The listing builds one solid part. Answer for the finished solid, in the listing's coordinates (mm). A direction names the side the tool comes from. Round coordinates to 2 decimals unless told otherwise and drop trailing zeros. Use a Markdown table: item, result. Add a question column.
1) Find the intervals of material crossed by probe 1 along X at (y, z) = (12, 7.75); probe 2 along X at (y, z) = (-13, 15); probe 3 along Y at (x, z) = (-18, 2.75), in increasing order. Write a range as from..to.
2) Determine the mould class of faces 5 (the flat face through (-38.04, -24.13, 2.87)), 6 (the flat face through (-0.2, 25.3, 20)), 7 (the flat face through (-11.64, 18.17, 9.86)) for opening direction Y: +Y half, -Y half, draft (parallel to the pull), parting line (faces both ways), or undercut.
3) A tool of negligible diameter and unlimited length cuts with its end or side. For faces 1 (the flat face through (-22.64, -8.02, 21.48)), 2 (the flat face through (0, -25.009, 10)), 3 (the flat face through (28, -5, 20)), 4 (the flat face through (16.98, -14.62, 21.48)), from which of +Z, -Z, +X, -X, +Y, -Y can it reach the whole face along a straight path? Write none if from no direction.
4) A cutting plane is placed at A-A (z = 8.75). State how many separate pieces and enclosed holes the cut face has, then the cut area to 3 significant figures.
5) Each of these flat-tipped pins is pushed along its axis until it touches: P1, Ø4, axis at y = -20, z = 9, coming from the +X side; P2, Ø6.5, axis at x = -3.5, y = -14, coming from the +Z side. Where does it stop, or does it pass through?
```python
from build123d import *

# Parameters (mm, degrees)
F1_DEPTH      = 20
F2_R          = 7
F3_DEPTH      = 98.6163846154
F3_DEPTH_BACK = 8.6163846154
F4_R          = 7
F5_DEPTH      = 98.6163846154
F5_DEPTH_BACK = 8.6163846154
F7_DEPTH      = 3
F8_T4_DEPTH   = 57.4298435113
F8_T9_DEPTH   = 57.4298435113
F8_T14_DEPTH  = 56.5459149398
F8_T19_DEPTH  = 56.5459149398
F8_T24_DEPTH  = 56.5459149398
F8_T29_DEPTH  = 56.5459149398
F8_T34_DEPTH  = 57.4298435113
F8_T39_DEPTH  = 57.4298435113
F9_T1_DEPTH   = 31.2168298797
F9_T3_DEPTH   = 31.2168298797
F9_T5_DEPTH   = 31.2168298797
F10_R         = 3


# Not quite as in the source:
# - a fillet or chamfer that OpenCascade refuses, or shapes differently, is made with other operations: its cross-section is extruded or revolved along the edge and cut away or added


with BuildPart() as f1:
    # F0 (on Top) → F1 (new body)
    with BuildSketch(Plane.XY):
        Polygon((-23.609552012, 25.0086836473), (0, 25.0086836473), (23.609552012, 25.0086836473), (34.109552012, 31.0086836473), (-34.109552012, 31.0086836473), align=None)
        Polygon((0, 11.517511069), (-23.609552012, 25.0086836473), (-34.109552012, 31.0086836473), (-44.0323307792, 13.6438208048), (-38.0323307792, 10.2152493762), (-20.1556443707, 0), align=None)
        Polygon((34.109552012, 31.0086836473), (23.609552012, 25.0086836473), (0, 11.517511069), (20.1556443707, 0), (38.0323307792, 10.2152493762), (44.0323307792, 13.6438208048), align=None)
        Polygon((-38.0323307792, 10.2152493762), (-44.0323307792, 13.6438208048), (-44.0323307792, -13.6438208048), (-38.0323307792, -10.2152493762), (-38.0323307792, 0), align=None)
        Polygon((0, -11.517511069), (-20.1556443707, 0), (-38.0323307792, -10.2152493762), (-44.0323307792, -13.6438208048), (-34.109552012, -31.0086836473), (-23.609552012, -25.0086836473), align=None)
        Polygon((38.0323307792, -10.2152493762), (20.1556443707, 0), (0, -11.517511069), (23.609552012, -25.0086836473), (34.109552012, -31.0086836473), (44.0323307792, -13.6438208048), align=None)
        Polygon((44.0323307792, -13.6438208048), (44.0323307792, 13.6438208048), (38.0323307792, 10.2152493762), (38.0323307792, 0), (38.0323307792, -10.2152493762), align=None)
        Polygon((-23.609552012, -25.0086836473), (-34.109552012, -31.0086836473), (34.109552012, -31.0086836473), (23.609552012, -25.0086836473), (0, -25.0086836473), align=None)
        Polygon((20.1556443707, 0), (0, 11.517511069), (-20.1556443707, 0), (0, -11.517511069), align=None)
    extrude(amount=F1_DEPTH)

    # F2 (on face) → F3 (cut, two sides)
    with BuildSketch(Plane(origin=(-39.0709413956, -22.3262522261, 0), x_dir=(0.4961389384, -0.8682431421, 0), z_dir=(-0.8682431421, -0.4961389384, 0))) as f3_sk:
        with Locations((0, 10)):
            Circle(F2_R)
    extrude(amount=-F3_DEPTH, mode=Mode.SUBTRACT)
    extrude(f3_sk.sketch, amount=F3_DEPTH_BACK, mode=Mode.SUBTRACT)

    # F4 (on face) → F5 (cut, two sides)
    with BuildSketch(Plane(origin=(39.0709413956, -22.3262522261, 0), x_dir=(0.4961389384, 0.8682431421, 0), z_dir=(0.8682431421, -0.4961389384, 0))) as f5_sk:
        with Locations((0, 10)):
            Circle(F4_R)
    extrude(amount=-F5_DEPTH, mode=Mode.SUBTRACT)
    extrude(f5_sk.sketch, amount=F5_DEPTH_BACK, mode=Mode.SUBTRACT)

    # F6 (on face) → F7 (join)
    with BuildSketch(Plane.XY.offset(20)):
        Polygon((0, 0.8638133302), (-38.6988371918, 22.9774345827), (-39.0709413956, 22.3262522261), (-39.4430455994, 21.6750698695), (-1.5116733278, 0), align=None)
        Polygon((38.6988371918, 22.9774345827), (0, 0.8638133302), (1.5116733278, 0), (39.4430455994, 21.6750698695), (39.0709413956, 22.3262522261), align=None)
        Polygon((1.5116733278, 0), (0, 0.8638133302), (-1.5116733278, 0), (0, -0.8638133302), align=None)
        Polygon((39.4430455994, -21.6750698695), (1.5116733278, 0), (0, -0.8638133302), (38.6988371918, -22.9774345827), (39.0709413956, -22.3262522261), align=None)
        Polygon((0, -0.8638133302), (-1.5116733278, 0), (-39.4430455994, -21.6750698695), (-39.0709413956, -22.3262522261), (-38.6988371918, -22.9774345827), align=None)
    extrude(amount=F7_DEPTH)

    # F8: chamfer of 5 on 8 edges, made by hand


with BuildPart() as f8_tool2:
    # F8_s3 → F8_t4 (new body)
    with BuildSketch(Plane(origin=(-39.0709413956, -22.3262522261, 0), x_dir=(0, 0, 1), z_dir=(0.8682431421, 0.4961389384, 0))):
        Polygon((20, 5.75), (25, 0.75), (20, 0.75), align=None)
    extrude(amount=F8_T4_DEPTH)

    split(bisect_by=Plane.XY.offset(23), keep=Keep.BOTTOM)


with BuildPart() as f1_1:
    add(f1.part)

    # F8_t1: union F8_tool2
    add(f8_tool2.part)


with BuildPart() as f8_tool7:
    # F8_s8 → F8_t9 (new body)
    with BuildSketch(Plane(origin=(-10.7921263863, 6.1669293636, 0), x_dir=(0, 0, 1), z_dir=(0.8682431421, -0.4961389384, 0))):
        Polygon((20, 5.75), (25, 0.75), (20, 0.75), align=None)
    extrude(amount=F8_T9_DEPTH)

    split(bisect_by=Plane.XY.offset(23), keep=Keep.BOTTOM)


with BuildPart() as f1_2:
    add(f1_1.part)

    # F8_t6: union F8_tool7
    add(f8_tool7.part)


with BuildPart() as f8_tool12:
    # F8_s13 → F8_t14 (new body)
    with BuildSketch(Plane(origin=(10.0246614661, 5.7283779806, 0), x_dir=(0, 0, 1), z_dir=(-0.8682431421, -0.4961389384, 0))):
        Polygon((20, 5.75), (25, 0.75), (20, 0.75), align=None)
    extrude(amount=F8_T14_DEPTH)

    split(bisect_by=Plane.XY.offset(23), keep=Keep.BOTTOM)


with BuildPart() as f1_3:
    add(f1_2.part)

    # F8_t11: union F8_tool12
    add(f8_tool12.part)


with BuildPart() as f8_tool17:
    # F8_s18 → F8_t19 (new body)
    with BuildSketch(Plane(origin=(-39.0709413956, 22.3262522261, 0), x_dir=(0, 0, 1), z_dir=(0.8682431421, -0.4961389384, 0))):
        Polygon((20, 5.75), (25, 0.75), (20, 0.75), align=None)
    extrude(amount=F8_T19_DEPTH)

    split(bisect_by=Plane.XY.offset(23), keep=Keep.BOTTOM)


with BuildPart() as f1_4:
    add(f1_3.part)

    # F8_t16: union F8_tool17
    add(f8_tool17.part)


with BuildPart() as f8_tool22:
    # F8_s23 → F8_t24 (new body)
    with BuildSketch(Plane(origin=(39.0709413956, -22.3262522261, 0), x_dir=(0, 0, 1), z_dir=(-0.8682431421, 0.4961389384, 0))):
        Polygon((20, 5.75), (25, 0.75), (20, 0.75), align=None)
    extrude(amount=F8_T24_DEPTH)

    split(bisect_by=Plane.XY.offset(23), keep=Keep.BOTTOM)


with BuildPart() as f1_5:
    add(f1_4.part)

    # F8_t21: union F8_tool22
    add(f8_tool22.part)


with BuildPart() as f8_tool27:
    # F8_s28 → F8_t29 (new body)
    with BuildSketch(Plane(origin=(-10.0246614661, -5.7283779806, 0), x_dir=(0, 0, 1), z_dir=(0.8682431421, 0.4961389384, 0))):
        Polygon((20, 5.75), (25, 0.75), (20, 0.75), align=None)
    extrude(amount=F8_T29_DEPTH)

    split(bisect_by=Plane.XY.offset(23), keep=Keep.BOTTOM)


with BuildPart() as f1_6:
    add(f1_5.part)

    # F8_t26: union F8_tool27
    add(f8_tool27.part)


with BuildPart() as f8_tool32:
    # F8_s33 → F8_t34 (new body)
    with BuildSketch(Plane(origin=(10.7921263863, -6.1669293636, 0), x_dir=(0, 0, 1), z_dir=(-0.8682431421, 0.4961389384, 0))):
        Polygon((20, 5.75), (25, 0.75), (20, 0.75), align=None)
    extrude(amount=F8_T34_DEPTH)

    split(bisect_by=Plane.XY.offset(23), keep=Keep.BOTTOM)


with BuildPart() as f1_7:
    add(f1_6.part)

    # F8_t31: union F8_tool32
    add(f8_tool32.part)


with BuildPart() as f8_tool37:
    # F8_s38 → F8_t39 (new body)
    with BuildSketch(Plane(origin=(39.0709413956, 22.3262522261, 0), x_dir=(0, 0, 1), z_dir=(-0.8682431421, -0.4961389384, 0))):
        Polygon((20, 5.75), (25, 0.75), (20, 0.75), align=None)
    extrude(amount=F8_T39_DEPTH)

    split(bisect_by=Plane.XY.offset(23), keep=Keep.BOTTOM)


with BuildPart() as f1_8:
    add(f1_7.part)

    # F8_t36: union F8_tool37
    add(f8_tool37.part)

    # F9: chamfer of 5 on 4 edges, made by hand

    # F9_s2 → F9_t1 (cut)
    with BuildSketch(Plane(origin=(7.7439424177, -13.5518992309, 0), x_dir=(0, 0, 1), z_dir=(-0.4961389384, 0.8682431421, 0))):
        Polygon((18, -45), (23, -40), (23, -45), align=None)
        Polygon((18, 45), (23, 40), (23, 45), align=None)
    extrude(amount=F9_T1_DEPTH, mode=Mode.SUBTRACT)

    # F9_s4 → F9_t3 (cut)
    with BuildSketch(Plane(origin=(7.7439424177, 13.5518992309, 0), x_dir=(0, 0, 1), z_dir=(-0.4961389384, -0.8682431421, 0))):
        Polygon((18, 45), (23, 40), (23, 45), align=None)
    extrude(amount=F9_T3_DEPTH, mode=Mode.SUBTRACT)

    # F9_s6 → F9_t5 (cut)
    with BuildSketch(Plane(origin=(-7.7439424177, -13.5518992309, 0), x_dir=(0, 0, 1), z_dir=(0.4961389384, 0.8682431421, 0))):
        Polygon((18, 45), (23, 40), (23, 45), align=None)
    extrude(amount=F9_T5_DEPTH, mode=Mode.SUBTRACT)

    # F10
    f10_edges = [f1_8.edges().sort_by_distance(p)[0] for p in [
        (0, 31.008684, 20),
        (0, -31.008684, 20),
        (-44.032331, 0, 20),
        (44.032331, 0, 20),
    ]]
    fillet(f10_edges, radius=F10_R)


solid = f1_8.part
```
Entries:
| question | item | result |
|---|---|---|
| 1 | probe 1 | x = -44.03..-34.36, -7.64..-0.84, 0.84..7.64, 34.36..44.03 |
| 1 | probe 2 | x = -44.03..-32.62, -12.88..-2.59, 2.59..12.88, 32.62..44.03 |
| 1 | probe 3 | y = -31.01..-25.01, -21.8..21.8, 25.01..31.01 |
| 2 | face 5 | -Y half |
| 2 | face 6 | draft |
| 2 | face 7 | undercut |
| 3 | face 1 | +Z, -X |
| 3 | face 2 | +Z, -Z |
| 3 | face 3 | +Z, +X |
| 3 | face 4 | +Z, -Y |
| 4 | separate pieces | 4 |
| 4 | enclosed holes | 4 |
| 4 | area | 1,860 mm² |
| 5 | P1 | stops at x = 24.61 |
| 5 | P2 | stops at z = 20 |
